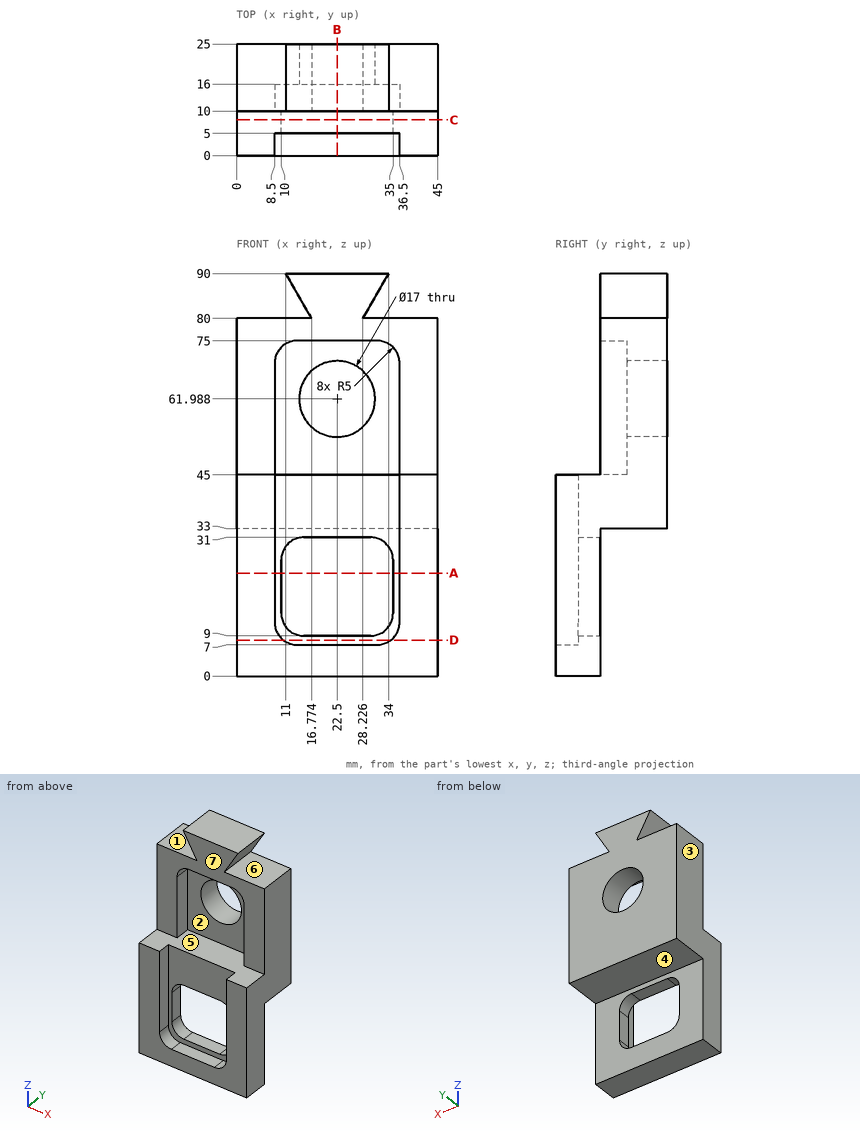
Answer from the drawing. Dimensions are ordinates in mm from the lowest x, y and z of the part. A direction names the side the tool comes from. Coordinates: 2 decimals unless noted, no trailing zeros. Order: outer loops, then holes, each group sorted by start corner. A loop starts at its lowest first (then second) coordinate and runs counter-clockwise, first axis right, second up. Notation, with made-up numbers: (17.25, 3) - (38.25, 3) arc R24 cw to (38.25, 27) - close; hole circle Ø3 at (44.25, -2.5). An arc over 180 degrees is marked (long way). Use one line per item in the form item = value.
(1) Straight lines are drawn through the part: L1, parallel to Z at x = 32.5, y = 10.75 (1 decimal); L2, parallel to Z at x = 22.5, y = 22; L3, parallel to X at y = 6, z = 25. For each, find the intervals that lie inside material, in ascending order.
Computed values:
L1 = 33 to 45, 74.9 to 80, 87.4 to 90
L2 = 33 to 53.49, 70.49 to 90
L3 = 0 to 10, 35 to 45
(2) For a pull along X with two mould halves and no side action, classify the marked faces 1, 2 and 3 as pulls with the +X half, pulls with the -X half, needs draft (parallel to the pull), parting line crosses it, or undercut.
Computed values:
face_1 = needs draft
face_2 = undercut
face_3 = pulls with the -X half
(3) Given pin 1 Ø12 at (x, y) = (30.5, 19) entering from -Z; pin 2 Ø16.5 at (x, z) = (20, 9.5) entering from +Y; pin 3 Ø22.5 at (x, z) = (23.5, 66) entering from -Y, each flat-ended and moving along its own axis, determine where each tip first touches the part or whether it passes through.
Computed values:
pin_1 = 33
pin_2 = 10
pin_3 = 10
(4) Section B-B, the plane x = 22.5 is taken. Give the vertices of the cut face in (y, z), then the cut area to 3 significant figures.
Computed values:
outline = (0, 0) - (10, 0) - (10, 9) - (5, 9) - (5, 7) - (0, 7) - close; (5, 31) - (10, 31) - (10, 33) - (25, 33) - (25, 53.49) - (16, 53.49) - (16, 45) - (5, 45) - close; (10, 75) - (16, 75) - (16, 70.49) - (25, 70.49) - (25, 90) - (10, 90) - close
area = 672 mm²
(5) Section D-D, the plane z = 8 is taken. Give the vertices of the cut face in (x, y).
Computed values:
outline = (0, 0) - (10.5, 0) - (10.5, 5) - (34.5, 5) - (34.5, 0) - (45, 0) - (45, 10) - (0, 10) - close
(6) Which of the six approach directions +Z, -Z, +X, -X, +Y, -Y give full straight-line access (tool end or side, diameter ignored) to the marked faces 4, 5, 6 and 7?
Computed values:
face_4 = -Z, +X, -X, +Y
face_5 = -Y
face_6 = +X, +Y, -Y
face_7 = +Z, +X, -X, -Y
(7) Section C-C, the plane y = 8 is taken. Give the vertices of the cut face in (x, z), then the cut area to 3 significant figures.
Computed values:
outline = (0, 0) - (45, 0) - (45, 45) - (0, 45) - close; hole (10, 14) arc R5 ccw to (15, 9) - (30, 9) arc R5 ccw to (35, 14) - (35, 26) arc R5 ccw to (30, 31) - (15, 31) arc R5 ccw to (10, 26) - close
area = 1,500 mm²
(8) Section A-A, the plane z = 23 is taken. Give the vertices of the cut face in (x, y).
Computed values:
outline = (0, 0) - (8.5, 0) - (8.5, 5) - (10, 5) - (10, 10) - (0, 10) - close; (35, 5) - (36.5, 5) - (36.5, 0) - (45, 0) - (45, 10) - (35, 10) - close
